Work out the finished part from the listing and answer in its coordinate system (mm). Face numbers are marked on the shaded views. A direction names the side the tool comes from. Give positions to 0.01 mm unless a question says otherwise; leave off trailing zeros. Loops run counter-clockwise (first coordinate to the right, second up) from the corner with the lowest first, then second, coordinate; pieces in that order, holes last. Notation, with made-up numbers: (-2.5, -17.75) - (5.5, -17.75) arc R11 ccw to (5.5, -11.75) - close; hole circle Ø7 at (-23, 26.25). An arc over 180 degrees is marked (long way). One line per item, written item: value.
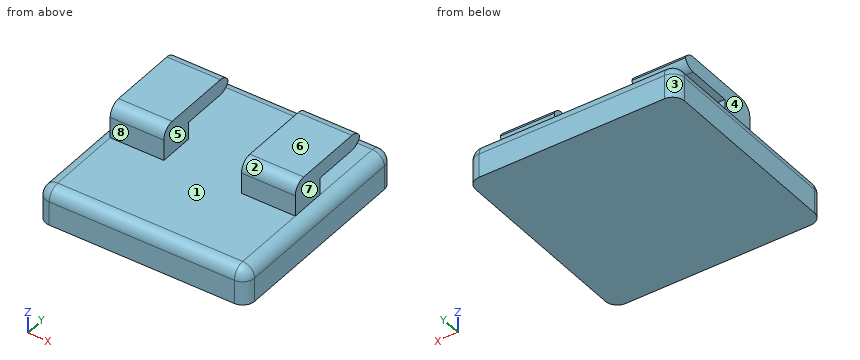
from build123d import *

# Parameters (mm, degrees)
BOSS_EXTRUDE1_DEPTH     = 44.45
CUT_EXTRUDE1_DEPTH      = 6.35
CUT_EXTRUDE1_DEPTH_BACK = 3.81
SKETCH2_W               = 2.54
SKETCH2_H               = 19.817543538
CUT_EXTRUDE2_DEPTH      = 5.08
CUT_EXTRUDE2_DEPTH_BACK = 3.81
SKETCH4_W               = 2.544966755
SKETCH4_H               = 19.817543538
CUT_EXTRUDE3_DEPTH      = 5.08
CUT_EXTRUDE3_DEPTH_BACK = 3.81
SKETCH8_W               = 16.513276495
SKETCH8_H               = 19.817543538
FILLET3_DEPTH           = 44.45
FILLET3_START           = 7
FILLET3_2_DEPTH         = 47
FILLET4_R               = 2.54
FILLET5_R               = 2.54
FILLET6_R               = 2.54


with BuildPart() as part:
    # Sketch1 → Boss-Extrude1 (new body)
    with BuildSketch(Plane(origin=(0, 0, 0), x_dir=(0, 0, -1), z_dir=(1, 0, 0))):
        Polygon((-4.141724441, 52.87490044), (-11.761724441, 52.87490044), (-11.761724441, 34.478280211), (-15.434687804, 34.478280211), (-15.434687804, 46.643996602), (-18.737279906, 46.643996602), (-18.737279906, 26.921380181), (-11.761724441, 26.921380181), (-11.761724441, 8.42490044), (-4.141724441, 8.42490044), align=None)
    extrude(amount=BOSS_EXTRUDE1_DEPTH)

    # Sketch2 → Cut-Extrude1 (cut, two sides: drawn at the far end of the back side and taken through both)
    with BuildSketch(Plane.XY.offset(15.571724441).offset(-CUT_EXTRUDE1_DEPTH_BACK)):
        with Locations((43.18, 36.735224833)):
            Rectangle(SKETCH2_W, SKETCH2_H)
    extrude(amount=CUT_EXTRUDE1_DEPTH + CUT_EXTRUDE1_DEPTH_BACK, mode=Mode.SUBTRACT)

    # Sketch4 → Cut-Extrude2 (cut, two sides: drawn at the far end of the back side and taken through both)
    with BuildSketch(Plane.XY.offset(15.571724441).offset(-CUT_EXTRUDE2_DEPTH_BACK)):
        with Locations((1.272483378, 36.735224833)):
            Rectangle(SKETCH4_W, SKETCH4_H)
    extrude(amount=CUT_EXTRUDE2_DEPTH + CUT_EXTRUDE2_DEPTH_BACK, mode=Mode.SUBTRACT)

    # Sketch8 → Cut-Extrude3 (cut, two sides: drawn at the far end of the back side and taken through both)
    with BuildSketch(Plane.XY.offset(15.571724441).offset(-CUT_EXTRUDE3_DEPTH_BACK)):
        with Locations((22.215391178, 36.735224833)):
            Rectangle(SKETCH8_W, SKETCH8_H)
    extrude(amount=CUT_EXTRUDE3_DEPTH + CUT_EXTRUDE3_DEPTH_BACK, mode=Mode.SUBTRACT)

    # Fillet3: read off the stored shape, not the designer's step
    # Fillet3 outline → Fillet3 (cut)
    with BuildSketch(Plane.YZ):
        with BuildLine():
            ThreePointArc((8.42490044, 9.221724441), (9.168849215, 11.017775666), (10.96490044, 11.761724441))
            Line((10.96490044, 11.761724441), (8.42490044, 11.761724441))
            Line((8.42490044, 11.761724441), (8.42490044, 9.221724441))
        make_face()
        with BuildLine():
            ThreePointArc((50.33490044, 11.761724441), (52.130951664, 11.017775665), (52.87490044, 9.221724441))
            Line((52.87490044, 9.221724441), (52.87490044, 11.761724441))
            Line((52.87490044, 11.761724441), (50.33490044, 11.761724441))
        make_face()
    extrude(amount=FILLET3_DEPTH, mode=Mode.SUBTRACT)

    # Fillet3 2 outline → Fillet3 2 (cut)
    with BuildSketch(Plane(origin=(0, 0, 0), x_dir=(1, 0, 0), z_dir=(0, 1, 0)).offset(FILLET3_START)):
        with BuildLine():
            Line((0, -11.761724441), (2.54, -11.761724441))
            ThreePointArc((2.54, -11.761724441), (0.743948776, -11.017775665), (0, -9.221724441))
            Line((0, -9.221724441), (0, -11.761724441))
        make_face()
        with BuildLine():
            ThreePointArc((44.45, -9.221724441), (43.706051224, -11.017775665), (41.91, -11.761724441))
            Line((41.91, -11.761724441), (44.45, -11.761724441))
            Line((44.45, -11.761724441), (44.45, -9.221724441))
        make_face()
    extrude(amount=FILLET3_2_DEPTH, mode=Mode.SUBTRACT)

    # Fillet4
    # the kernel refuses this fillet: 2.54 mm, written as the material it takes off along each edge
    with BuildSketch(Plane(origin=(41.91, 50.33490044, 9.221724441), x_dir=(1, 0, 0), z_dir=(0, 1, 0))) as fillet4_piece_1_section:
        Polygon((0, 0), (FILLET4_R, 0), (FILLET4_R, -FILLET4_R), (0, -FILLET4_R), align=None)
    fillet4_piece_1 = extrude(amount=FILLET4_R, mode=Mode.PRIVATE)
    fillet4_piece_1 = fillet4_piece_1 - Plane(origin=(41.91, 50.33490044, 9.221724441), x_dir=(-0.7071067811865475, 0, -0.7071067811865475), z_dir=(0, 1, 0)) * Sphere(FILLET4_R, mode=Mode.PRIVATE)
    add(fillet4_piece_1, mode=Mode.SUBTRACT)
    with BuildSketch(Plane(origin=(2.54, 50.33490044, 9.221724441), x_dir=(-1, 0, 0), z_dir=(0, 1, 0))) as fillet4_piece_2_section:
        Polygon((0, 0), (FILLET4_R, 0), (FILLET4_R, FILLET4_R), (0, FILLET4_R), align=None)
    fillet4_piece_2 = extrude(amount=FILLET4_R, mode=Mode.PRIVATE)
    fillet4_piece_2 = fillet4_piece_2 - Plane(origin=(2.54, 50.33490044, 9.221724441), x_dir=(0.7071067811865475, 0, -0.7071067811865475), z_dir=(0, 1, 0)) * Sphere(FILLET4_R, mode=Mode.PRIVATE)
    add(fillet4_piece_2, mode=Mode.SUBTRACT)
    with BuildSketch(Plane(origin=(41.91, 10.96490044, 9.221724441), x_dir=(0, -1, 0), z_dir=(1, 0, 0))) as fillet4_piece_3_section:
        Polygon((0, 0), (FILLET4_R, 0), (FILLET4_R, -FILLET4_R), (0, -FILLET4_R), align=None)
    fillet4_piece_3 = extrude(amount=FILLET4_R, mode=Mode.PRIVATE)
    fillet4_piece_3 = fillet4_piece_3 - Plane(origin=(41.91, 10.96490044, 9.221724441), x_dir=(0, 0.7071067811865476, -0.7071067811865475), z_dir=(1, 0, 0)) * Sphere(FILLET4_R, mode=Mode.PRIVATE)
    add(fillet4_piece_3, mode=Mode.SUBTRACT)
    with BuildSketch(Plane(origin=(2.54, 10.96490044, 9.221724441), x_dir=(0, -1, 0), z_dir=(-1, 0, 0))) as fillet4_piece_4_section:
        Polygon((0, 0), (FILLET4_R, 0), (FILLET4_R, FILLET4_R), (0, FILLET4_R), align=None)
    fillet4_piece_4 = extrude(amount=FILLET4_R, mode=Mode.PRIVATE)
    fillet4_piece_4 = fillet4_piece_4 - Plane(origin=(2.54, 10.96490044, 9.221724441), x_dir=(0, 0.7071067811865476, -0.7071067811865475), z_dir=(-1, 0, 0)) * Sphere(FILLET4_R, mode=Mode.PRIVATE)
    add(fillet4_piece_4, mode=Mode.SUBTRACT)
    with BuildSketch(Plane(origin=(0, 52.87490044, -2.208275559), x_dir=(1, 0, 0), z_dir=(0, 0, 1)), Plane(origin=(44.45, 8.42490044, 9.221724441), x_dir=(0, 1, 0), z_dir=(0, 0, -1))) as fillet4_piece_5:
        with BuildLine():
            CenterArc((FILLET4_R, -FILLET4_R), FILLET4_R, 90, 90)
            Line((0, -FILLET4_R), (0, 0))
            Line((0, 0), (FILLET4_R, 0))
        make_face()
    extrude(amount=11.43, mode=Mode.SUBTRACT)
    with BuildSketch(Plane(origin=(44.45, 52.87490044, -2.208275559), x_dir=(-1, 0, 0), z_dir=(0, 0, 1)), Plane(origin=(0, 8.42490044, 9.221724441), x_dir=(0, 1, 0), z_dir=(0, 0, -1))) as fillet4_piece_6:
        with BuildLine():
            CenterArc((FILLET4_R, FILLET4_R), FILLET4_R, 180, 90)
            Line((0, FILLET4_R), (0, 0))
            Line((0, 0), (FILLET4_R, 0))
        make_face()
    extrude(amount=11.43, mode=Mode.SUBTRACT)

    # Fillet5
    # the kernel refuses this fillet: 2.54 mm, written as the material it takes off along each edge
    with BuildSketch(Plane(origin=(24.122029425, 46.643996602, 18.737279906), x_dir=(0, -1, 0), z_dir=(1, 0, 0)), Plane(origin=(24.122029425, 46.643996602, 15.434687804), x_dir=(0, 0, 1), z_dir=(1, 0, 0))) as fillet5_piece_1:
        with BuildLine():
            CenterArc((FILLET5_R, FILLET5_R), FILLET5_R, 180, 90)
            Line((0, FILLET5_R), (0, 0))
            Line((0, 0), (FILLET5_R, 0))
        make_face()
    extrude(amount=24.137970575, mode=Mode.SUBTRACT)
    with BuildSketch(Plane(origin=(-3.805033245, 46.643996602, 18.737279906), x_dir=(0, 0, -1), z_dir=(1, 0, 0)), Plane(origin=(-3.805033245, 46.643996602, 15.434687804), x_dir=(0, -1, 0), z_dir=(1, 0, 0))) as fillet5_piece_2:
        with BuildLine():
            CenterArc((FILLET5_R, -FILLET5_R), FILLET5_R, 90, 90)
            Line((0, -FILLET5_R), (0, 0))
            Line((0, 0), (FILLET5_R, 0))
        make_face()
    extrude(amount=24.113786175, mode=Mode.SUBTRACT)

    # Fillet6
    fillet6_edges = [part.edges().sort_by_distance(p)[0] for p in [
        (36.191014713, 26.921380181, 18.737279906),
        (8.251859842, 26.921380181, 18.737279906),
    ]]
    fillet(fillet6_edges, radius=FILLET6_R)


solid = part.part
1. Section A-A (y = 39) is taken. Write down the section's boundary in (x, z).
Output:
outline: (0, 4.14) - (44.45, 4.14) - (44.45, 9.22) arc R2.54 ccw to (41.91, 11.76) - (2.54, 11.76) arc R2.54 ccw to (0, 9.22) - close; (2.54, 15.43) - (13.96, 15.43) - (13.96, 18.74) - (2.54, 18.74) - close; (30.47, 15.43) - (41.91, 15.43) - (41.91, 18.74) - (30.47, 18.74) - close
2. The mould has two halves that part along Z. Classify the marked faces 1, 2 and 3: released by +Z, released by -Z, zero draft, split by the parting line, or undercut.
Output:
face 1: undercut
face 2: released by +Z
face 3: zero draft
3. Section B-B (z = 12.75) is taken. Write down the section's boundary in (x, y).
Output:
outline: (2.54, 26.92) - (13.96, 26.92) - (13.96, 34.48) - (2.54, 34.48) - close; (30.47, 26.92) - (41.91, 26.92) - (41.91, 34.48) - (30.47, 34.48) - close
4. Find the intervals of material crossed by line 1 along Z through (x, y) = (33.5, 39.5); line 2 along X through (y, z) = (38, 17); line 3 along Y through (x, z) = (12.5, 15), in increasing order.
Output:
line 1: z = 4.14 to 11.76, 15.43 to 18.74
line 2: x = 2.54 to 13.96, 30.47 to 41.91
line 3: y = 26.92 to 34.48
5. Section D-D (y = 16) is taken. Write down the section's boundary in (x, z).
Output:
outline: (0, 4.14) - (44.45, 4.14) - (44.45, 9.22) arc R2.54 ccw to (41.91, 11.76) - (2.54, 11.76) arc R2.54 ccw to (0, 9.22) - close
6. Section C-C (x = 36) is taken. Write down the section's boundary in (y, z).
Output:
outline: (8.42, 4.14) - (52.87, 4.14) - (52.87, 9.22) arc R2.54 ccw to (50.33, 11.76) - (34.48, 11.76) - (34.48, 15.43) - (44.1, 15.43) arc R2.54 ccw to (46.48, 17.09) arc R2.54 ccw to (44.1, 18.74) - (29.46, 18.74) arc R2.54 ccw to (26.92, 16.2) - (26.92, 11.76) - (10.96, 11.76) arc R2.54 ccw to (8.42, 9.22) - close
7. Flat-ended cylindrical pins translate along their axes: pin 1 Ø8 at (x, z) = (16.5, 15.5) entering from +Y; pin 2 Ø6 at (y, z) = (46.5, 16) entering from +X; pin 3 Ø5 at (y, z) = (47, 14) entering from +X. Find the tip coordinate at first contact, or state that the pin passes through.
Output:
pin 1: stops at y = 51.46
pin 2: stops at x = 41.91
pin 3: stops at x = 43.03
8. For the marked faces 4, 5, 6, 7 and 8, determine the directions among +Z, -Z, +X, -X, +Y, -Y from which every point of the face is accessible in a straight line to the end or side of a thin tool.
Output:
face 4: +Z, -X, +Y, -Y
face 5: +Z, +Y, -Y
face 6: +Z, +X, -X, +Y, -Y
face 7: +Z, +X, +Y, -Y
face 8: +Z, +X, -X, -Y
